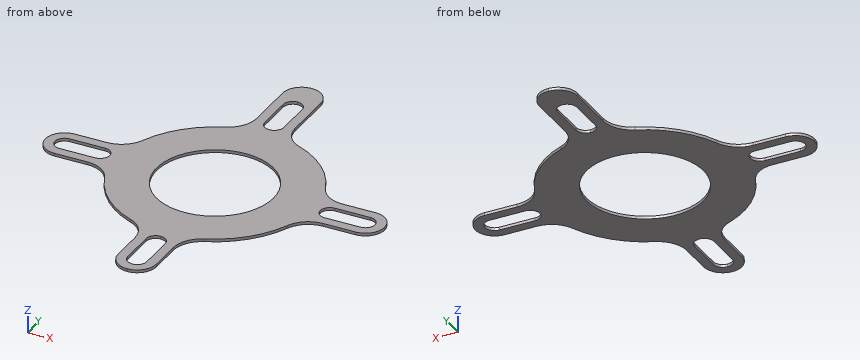
from build123d import *

# Parameters (mm, degrees)
F0_R     = 30.5
F0_W     = 5
F0_H     = 10.5
F0_W_2   = 10.5
F0_H_2   = 5
F1_DEPTH = 1.5


# Not quite as in the source:
# - a feature names something its author has since deleted; it is built from what else it names


with BuildPart() as f1:
    # F0 (on Top) → F1 (new body)
    with BuildSketch(Plane.XY):
        with BuildLine():
            ThreePointArc((-10, 61.6218305473), (-12.5584071324, 53.2428827066), (-19.3609022556, 47.7221695216))
            ThreePointArc((-19.3609022556, 47.7221695216), (-36.4159992311, 36.4159992311), (-47.7221695216, 19.3609022556))
            ThreePointArc((-47.7221695216, 19.3609022556), (-53.2428827066, 12.5584071324), (-61.6218305473, 10))
            Line((-61.6218305473, 10), (-65.6218305473, 10))
            Line((-65.6218305473, 10), (-65.6218305473, 5))
            Line((-65.6218305473, 5), (-59.986856736, 5))
            ThreePointArc((-59.986856736, 5), (-56.45132283, 3.5355339059), (-54.986856736, 0))
            ThreePointArc((-54.986856736, 0), (-56.45132283, -3.5355339059), (-59.986856736, -5))
            Line((-59.986856736, -5), (-65.6218305473, -5))
            Line((-65.6218305473, -5), (-65.6218305473, -10))
            Line((-65.6218305473, -10), (-61.6218305473, -10))
            ThreePointArc((-61.6218305473, -10), (-53.2428827066, -12.5584071324), (-47.7221695216, -19.3609022556))
            ThreePointArc((-47.7221695216, -19.3609022556), (-36.4159992311, -36.4159992311), (-19.3609022556, -47.7221695216))
            ThreePointArc((-19.3609022556, -47.7221695216), (-12.5584071324, -53.2428827066), (-10, -61.6218305473))
            Line((-10, -61.6218305473), (-10, -65.6218305473))
            Line((-10, -65.6218305473), (-5, -65.6218305473))
            Line((-5, -65.6218305473), (-5, -59.986856736))
            ThreePointArc((-5, -59.986856736), (-3.5355339059, -56.45132283), (0, -54.986856736))
            ThreePointArc((0, -54.986856736), (3.5355339059, -56.45132283), (5, -59.986856736))
            Line((5, -59.986856736), (5, -65.6218305473))
            Line((5, -65.6218305473), (10, -65.6218305473))
            Line((10, -65.6218305473), (10, -61.6218305473))
            ThreePointArc((10, -61.6218305473), (12.5584071324, -53.2428827066), (19.3609022556, -47.7221695216))
            ThreePointArc((19.3609022556, -47.7221695216), (36.4159992311, -36.4159992311), (47.7221695216, -19.3609022556))
            ThreePointArc((47.7221695216, -19.3609022556), (53.2428827066, -12.5584071324), (61.6218305473, -10))
            Line((61.6218305473, -10), (65.6218305473, -10))
            Line((65.6218305473, -10), (65.6218305473, -5))
            Line((65.6218305473, -5), (59.986856736, -5))
            ThreePointArc((59.986856736, -5), (56.45132283, -3.5355339059), (54.986856736, 0))
            ThreePointArc((54.986856736, 0), (56.45132283, 3.5355339059), (59.986856736, 5))
            Line((59.986856736, 5), (65.6218305473, 5))
            Line((65.6218305473, 5), (65.6218305473, 10))
            Line((65.6218305473, 10), (61.6218305473, 10))
            ThreePointArc((61.6218305473, 10), (53.2428827066, 12.5584071324), (47.7221695216, 19.3609022556))
            ThreePointArc((47.7221695216, 19.3609022556), (36.4159992311, 36.4159992311), (19.3609022556, 47.7221695216))
            ThreePointArc((19.3609022556, 47.7221695216), (12.5584071324, 53.2428827066), (10, 61.6218305473))
            Line((10, 61.6218305473), (10, 65.6218305473))
            Line((10, 65.6218305473), (5, 65.6218305473))
            Line((5, 65.6218305473), (5, 59.986856736))
            ThreePointArc((5, 59.986856736), (3.5355339059, 56.45132283), (0, 54.986856736))
            ThreePointArc((0, 54.986856736), (-3.5355339059, 56.45132283), (-5, 59.986856736))
            Line((-5, 59.986856736), (-5, 65.6218305473))
            Line((-5, 65.6218305473), (-10, 65.6218305473))
            Line((-10, 65.6218305473), (-10, 61.6218305473))
        make_face()
        Circle(F0_R, mode=Mode.SUBTRACT)
        with Locations((7.5, 70.8718305473)):
            Rectangle(F0_W, F0_H)
        with Locations((-7.5, 70.8718305473)):
            Rectangle(F0_W, F0_H)
        with Locations((70.8718305473, 7.5)):
            Rectangle(F0_W_2, F0_H_2)
        with Locations((70.8718305473, -7.5)):
            Rectangle(F0_W_2, F0_H_2)
        with BuildLine():
            Line((78.6218305473, 10), (76.1218305473, 10))
            Line((76.1218305473, 10), (76.1218305473, 5))
            Line((76.1218305473, 5), (78.6218305473, 5))
            ThreePointArc((78.6218305473, 5), (82.1573644532, 3.5355339059), (83.6218305473, 0))
            ThreePointArc((83.6218305473, 0), (82.1573644532, -3.5355339059), (78.6218305473, -5))
            Line((78.6218305473, -5), (76.1218305473, -5))
            Line((76.1218305473, -5), (76.1218305473, -10))
            Line((76.1218305473, -10), (78.6218305473, -10))
            ThreePointArc((78.6218305473, -10), (85.6928983592, -7.0710678119), (88.6218305473, 0))
            ThreePointArc((88.6218305473, 0), (85.6928983592, 7.0710678119), (78.6218305473, 10))
        make_face()
        with Locations((-70.8718305473, -7.5)):
            Rectangle(F0_W_2, F0_H_2)
        with Locations((-70.8718305473, 7.5)):
            Rectangle(F0_W_2, F0_H_2)
        with BuildLine():
            Line((-76.1218305473, 5), (-76.1218305473, 10))
            Line((-76.1218305473, 10), (-78.611907205, 10))
            ThreePointArc((-78.611907205, 10), (-85.6829750169, 7.0710678119), (-88.611907205, 0))
            ThreePointArc((-88.611907205, 0), (-85.6829750169, -7.0710678119), (-78.611907205, -10))
            Line((-78.611907205, -10), (-76.1218305473, -10))
            Line((-76.1218305473, -10), (-76.1218305473, -5))
            Line((-76.1218305473, -5), (-78.6218305473, -5))
            ThreePointArc((-78.6218305473, -5), (-82.1573644532, -3.5355339059), (-83.6218305473, 0))
            ThreePointArc((-83.6218305473, 0), (-82.1573644532, 3.5355339059), (-78.6218305473, 5))
            Line((-78.6218305473, 5), (-76.1218305473, 5))
        make_face()
        with Locations((-7.5, -70.8718305473)):
            Rectangle(F0_W, F0_H)
        with Locations((7.5, -70.8718305473)):
            Rectangle(F0_W, F0_H)
        with BuildLine():
            Line((-5, -76.1218305473), (-10, -76.1218305473))
            Line((-10, -76.1218305473), (-10, -78.611907205))
            ThreePointArc((-10, -78.611907205), (-7.0710678119, -85.6829750169), (0, -88.611907205))
            ThreePointArc((0, -88.611907205), (7.0710678119, -85.6829750169), (10, -78.611907205))
            Line((10, -78.611907205), (10, -76.1218305473))
            Line((10, -76.1218305473), (5, -76.1218305473))
            Line((5, -76.1218305473), (5, -78.6218305473))
            ThreePointArc((5, -78.6218305473), (3.5355339059, -82.1573644532), (0, -83.6218305473))
            ThreePointArc((0, -83.6218305473), (-3.5355339059, -82.1573644532), (-5, -78.6218305473))
            Line((-5, -78.6218305473), (-5, -76.1218305473))
        make_face()
        with BuildLine():
            Line((-10, 87.6788190633), (-10, 76.1218305473))
            Line((-10, 76.1218305473), (-5, 76.1218305473))
            Line((-5, 76.1218305473), (-5, 78.6218305473))
            ThreePointArc((-5, 78.6218305473), (-3.5355339059, 82.1573644532), (0, 83.6218305473))
            ThreePointArc((0, 83.6218305473), (3.5355339059, 82.1573644532), (5, 78.6218305473))
            Line((5, 78.6218305473), (5, 76.1218305473))
            Line((5, 76.1218305473), (10, 76.1218305473))
            Line((10, 76.1218305473), (10, 87.6788190633))
            ThreePointArc((10, 87.6788190633), (7.0710678119, 94.7498868751), (0, 97.6788190633))
            ThreePointArc((0, 97.6788190633), (-7.0710678119, 94.7498868751), (-10, 87.6788190633))
        make_face()
    extrude(amount=F1_DEPTH)


solid = f1.part
Verification items for the finished model (mm, model axes). Round coordinates to 2 decimals unless told otherwise and drop trailing zeros. Loops run counter-clockwise (first coordinate to the right, second up) from the corner with the lowest first, then second, coordinate; pieces in that order, holes last. Notation, with made-up numbers: (-37.5, -34) - (-19.5, -34) arc R9 ccw to (-19.5, -18) - close; hole circle Ø5 at (42.25, -5.75). An arc over 180 degrees is marked (long way). Write item = value, one per line.
Q1. Depth check by flat-ended pin: pin 1 (0.8 mm diameter, centred on x = -73.5, z = 0.5, fed in from -Y); pin 2 (0.8 mm diameter, centred on y = 79.5, z = 0.5, fed in from -X). Enter the tip coordinate at first touch or a pass-through.
Here are the results:
pin_1 = -10
pin_2 = -10
Q2. Sectioned sample at A-A on x = 66. Record the boundary of the cut face in (y, z).
Here are the results:
outline = (-10, 0) - (-5, 0) - (-5, 1.5) - (-10, 1.5) - close; (5, 0) - (10, 0) - (10, 1.5) - (5, 1.5) - close
Q3. Material ranges on L1, parallel to X at y = -78, z = 0.5; L2, parallel to Y at x = 61, z = 0.15; L3, parallel to X at y = 8.5, z = 1.05, recorded low to high.
Here are the results:
L1 = -10 to -5, 5 to 10
L2 = -10.01 to -5, 5 to 10.01
L3 = -83.88 to -29.29, 29.29 to 83.89
Q4. Sectioned sample at C-C on z = 0.4. State how many separate pieces and enclosed holes the cut face has, plus the area to 3 significant figures.
Here are the results:
separate_pieces = 1
enclosed_holes = 5
area = 7,530 mm^2
